```python
from build123d import *

# Parameters (mm, degrees)
F0_R            = 31.75
F1_DEPTH        = 12.7
F3_R            = 6.096
F4_DEPTH        = 25.4
F5_R            = 2.921
F6_DEPTH        = 19.05
F6_COPIES_COUNT = 8
F9_R            = 12.7
F10_DEPTH       = 101.6


# Not quite as in the source:
# - a pattern or mirror of a feature is missing from the dataset's text; its kind, count and spacing are read off the source's solid
# - the program builds the solid bodies; features that only make, move or delete a surface that nothing else refers to are left out


with BuildPart() as f1:
    # F0 (on Front) → F1 (new body)
    with BuildSketch(Plane.XZ):
        Circle(F0_R)
    extrude(amount=F1_DEPTH)

    # F3 (on face) → F4 (join)
    with BuildSketch(Plane.XZ.offset(12.7)):
        Circle(F3_R)
    extrude(amount=F4_DEPTH)

    # F5 (on face) → F6 (join)
    with BuildSketch(Plane.XZ.offset(12.7)):
        with Locations((5.1418263465, 22.225)):
            Circle(F5_R)
    f6 = extrude(amount=F6_DEPTH)

    # F6_copies: F6 ×8 about axis
    f6_copies_axis = Axis((0, 0, 0), (0, 1, 0))
    for i in range(1, F6_COPIES_COUNT):
        add(f6.rotate(f6_copies_axis, i * 360 / F6_COPIES_COUNT))

    # F9 (on face) → F10 (join)
    with BuildSketch(Plane(origin=(0, 0, 0), x_dir=(-1, 0, 0), z_dir=(0, 1, 0))):
        Circle(F9_R)
    extrude(amount=F10_DEPTH)


solid = f1.part
```
Here's how the part is built. I have some questions about the finished solid (model axes, mm). A direction names the side the tool comes from. Round coordinates to 2 decimals unless told otherwise and drop trailing zeros. Loops run counter-clockwise (first coordinate to the right, second up) from the corner with the lowest first, then second, coordinate; pieces in that order, holes last. Notation, with made-up numbers: (73.5, 83.25) -> (119.5, 83.25) arc R23 cw to (119.5, 110.25) -> close; hole circle Ø6 at (87, 77). An arc over 180 degrees is marked (long way). Answer as CSV lines item,"result". Start each with the question number.
1. Imagine slicing it at D-D on z = 27.5. Write out the boundary of the cut face in (x, y), plus the area to 3 significant figures.
2. Imagine slicing it at C-C on y = 76. Write out the boundary of the cut face in (x, z).
3. I need wall thicknesses on probe 1 along Y at (x, z) = (25, -15.5); probe 2 along Y at (x, z) = (4.5, 7.5); probe 3 along X at (y, z) = (-4, 14). Which ranges of each line are inside material? Lowest first, please. Write a range as from..to.
4. I'm going to push flat-ended pins straight in: P1, Ø6.5, axis at x = -5.5, z = -22.5, coming from the -Y side; P2, Ø3, axis at y = 24, z = -9.5, coming from the +X side; P3, Ø3, axis at y = 56.5, z = -8, coming from the +X side. Where does each tip first touch, or does it pass through?
5. Imagine slicing it at A-A on z = 0. Write out the boundary of the cut face in (x, y), plus the area to 3 significant figures.
6. Imagine slicing it at B-B on x = 0. Write out the boundary of the cut face in (y, z).
7. For faces 4 (the face through (-5, -31.75, -22)), 5 (the face through (20.45, -22.09, -2.82)), 6 (the face through (-22, -31.75, 5)), 7 (the face through (5, -31.75, 22)), which set-ups out of +Z, -Z, +X, -X, +Y, -Y let a thin tool reach every point of the face, with its end or its side?
8. If we mould it in two halves opening along Z, with no side actions, what happens to faces 1 (the face through (2.75, 50.09, -12.4)), 2 (the face through (-23.1, -22.09, 7.93)), 3 (the face through (-19, -31.75, -12))? For each: pulls with the +Z half, pulls with the -Z half, needs draft (parallel to the pull), parting line crosses it, or undercut.
Solution:
1,outline,"(-15.87, -12.7) -> (15.87, -12.7) -> (15.87, 0) -> (-15.87, 0) -> close"
1,area,"403 mm²"
2,outline,"circle Ø25.4 at (0, 0)"
3,probe 1,"-12.7..0"
3,probe 2,"-12.7..101.6"
3,probe 3,"-28.5..28.5"
4,P1,"y = -31.75"
4,P2,"x = 9.86"
4,P3,"x = 10.91"
5,outline,"(-31.75, -12.7) -> (-6.1, -12.7) -> (-6.1, -38.1) -> (6.1, -38.1) -> (6.1, -12.7) -> (31.75, -12.7) -> (31.75, 0) -> (12.7, 0) -> (12.7, 101.6) -> (-12.7, 101.6) -> (-12.7, 0) -> (-31.75, 0) -> close"
5,area,"3,700 mm²"
6,outline,"(-38.1, -6.1) -> (-12.7, -6.1) -> (-12.7, -31.75) -> (0, -31.75) -> (0, -12.7) -> (101.6, -12.7) -> (101.6, 12.7) -> (0, 12.7) -> (0, 31.75) -> (-12.7, 31.75) -> (-12.7, 6.1) -> (-38.1, 6.1) -> close"
7,face 4,"-Z, +X, -X, -Y"
7,face 5,"-Y"
7,face 6,"+Z, -Z, -X, -Y"
7,face 7,"+Z, +X, -X, -Y"
8,face 1,"parting line crosses it"
8,face 2,"undercut"
8,face 3,"needs draft"
